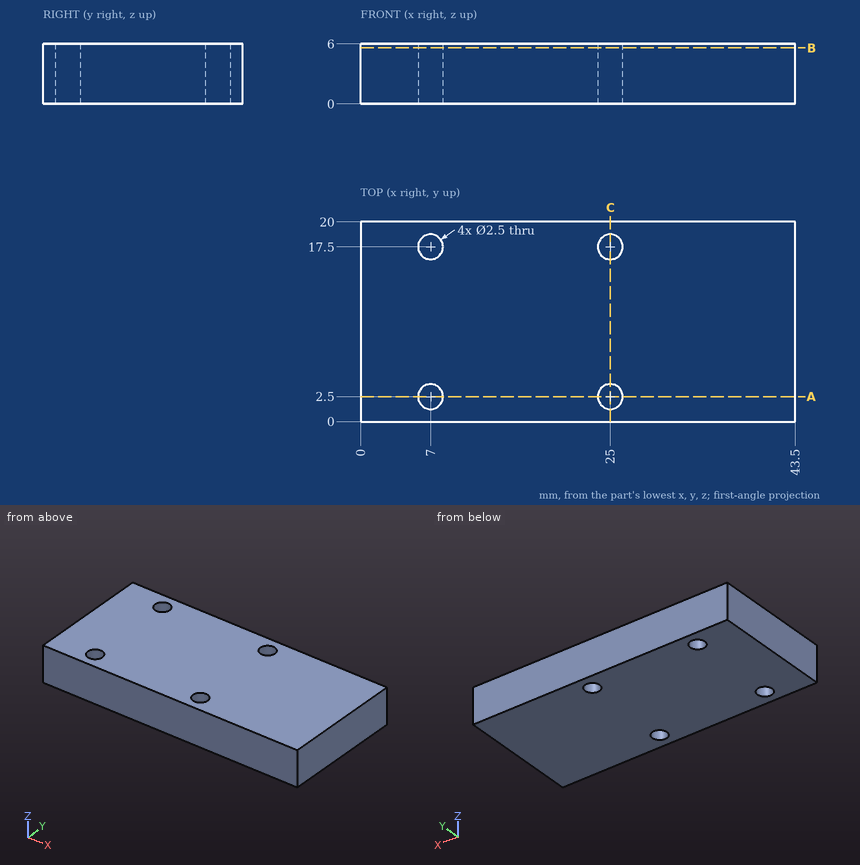
Geometry check sheet. Reference: drawing and pictorial views, mm from the part's lowest x, y, z. Coordinates: 2 decimals unless noted, no trailing zeros. Order: outer loops, then holes, each group sorted by start corner. A loop starts at its lowest first (then second) coordinate and runs counter-clockwise, first axis right, second up.
Item 1: Section check A-A, the plane y = 2.5. Enter the section's corners in (x, z).
Filled in:
outline: (0, 0) - (5.75, 0) - (5.75, 6) - (0, 6) - close; (8.25, 0) - (23.75, 0) - (23.75, 6) - (8.25, 6) - close; (26.25, 0) - (43.5, 0) - (43.5, 6) - (26.25, 6) - close
Item 2: Section check C-C, the plane x = 25. Enter the section's corners in (y, z), then the cut area to 3 significant figures.
Filled in:
outline: (0, 0) - (1.25, 0) - (1.25, 6) - (0, 6) - close; (3.75, 0) - (16.25, 0) - (16.25, 6) - (3.75, 6) - close; (18.75, 0) - (20, 0) - (20, 6) - (18.75, 6) - close
area: 90.0 mm2
Item 3: Section check B-B, the plane z = 5.6. Enter the section's corners in (x, y).
Filled in:
outline: (0, 0) - (43.5, 0) - (43.5, 20) - (0, 20) - close; hole circle Ø2.5 at (7, 2.5); hole circle Ø2.5 at (7, 17.5); hole circle Ø2.5 at (25, 2.5); hole circle Ø2.5 at (25, 17.5)
Item 4: Depth check by flat-ended pin: pin 1 (2 mm diameter, centred on x = 7, y = 2.5, fed in from -Z). Enter the tip coordinate at first touch or a pass-through.
Filled in:
pin 1: passes through
Item 5: Material ranges on L1, parallel to Y at x = 25, z = 3.9; L2, parallel to Y at x = 26, z = 1.1; L3, parallel to X at y = 16.75, z = 1.95, recorded low to high.
Filled in:
L1: y = 0 to 1.25, 3.75 to 16.25, 18.75 to 20
L2: y = 0 to 1.75, 3.25 to 16.75, 18.25 to 20
L3: x = 0 to 6, 8 to 24, 26 to 43.5
